Check sheet for the modelled part. Datum: model origin and axes. Units: mm. Face numbers are marked on the shaded views. A direction names the side the tool comes from. Give positions to 0.01 mm unless a question says otherwise; leave off trailing zeros. Order: outer loops, then holes, each group sorted by start corner. A loop starts at its lowest first (then second) coordinate and runs counter-clockwise, first axis right, second up.
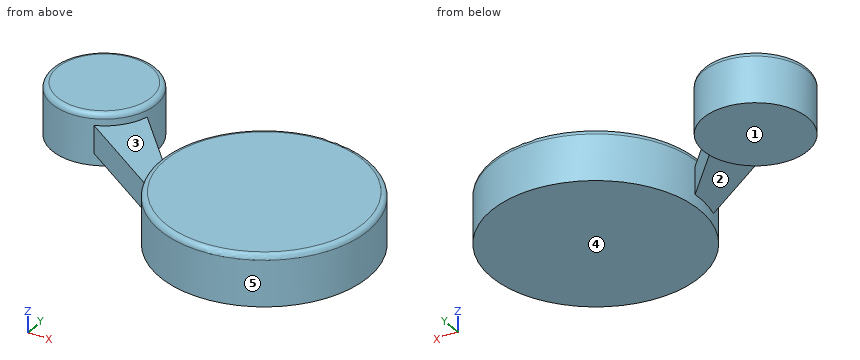
```python
from build123d import *

# Parameters (mm, degrees)
F0_R     = 101.6
F0_R_2   = 50.8
F1_DEPTH = 25
F2_R     = 5.08
F4_DEPTH = 13.5


with BuildPart() as f1:
    # F0 (on Top) → F1 (new body, symmetric)
    with BuildSketch(Plane.XY):
        with Locations((204.801934, 0)):
            Circle(F0_R)
        with Locations((0, 80.350283)):
            Circle(F0_R_2)
    extrude(amount=F1_DEPTH, both=True)

    # F2
    f2_edges = [f1.edges().sort_by_distance(p)[0] for p in [
        (-50.8, 80.350283, 25),
        (103.201934, 0, 25),
    ]]
    fillet(f2_edges, radius=F2_R)

    # F3 (on Top) → F4 (join, symmetric)
    with BuildSketch(Plane.XY):
        Polygon((10.487304, 110.720679), (17.449906, 34.354378), (178.083748, -74.550241), align=None)
    extrude(amount=F4_DEPTH, both=True)


solid = f1.part
```
(1) Cross-section at B-B on z = 6. Enter the section's corners in (x, y), then the cut area to 3 significant figures.
Response values:
outline: (19.06, 33.26) - (106.61, -26.09) arc R101.6 ccw (long way) to (103.51, 7.89) - (49.24, 67.88) arc R50.8 ccw (long way) to start
area: 43,600 mm2
(2) Cross-section at C-C on y = 0. Enter the section's corners in (x, z).
Response values:
outline: (68.12, -13.5) - (103.2, -13.5) - (103.2, -25) - (306.4, -25) - (306.4, 19.92) arc R5.08 ccw to (301.32, 25) - (108.28, 25) arc R5.08 ccw to (103.2, 19.92) - (103.2, 13.5) - (68.12, 13.5) - close
(3) Material ranges on L1, parallel to X at y = 89, z = -6; L2, parallel to Z at x = 77, y = -4; L3, parallel to X at y = 34.5, z = 11.5, recorded low to high.
Response values:
L1: x = -50.06 to 50.06, 155.8 to 253.81
L2: z = -13.5 to 13.5
L3: x = -21.87 to 79.44, 109.24 to 300.37
(4) Cross-section at D-D on z = -21. Enter the section's corners in (x, y).
Response values:
outline: circle Ø101.6 at (0, 80.35); circle Ø203.2 at (204.8, 0)
(5) Gauge pin test, flat ends, axial feed: pin 1 Ø3 at (y, z) = (76.5, 14.5) entering from +X; pin 2 Ø1 at (y, z) = (-5, -0.5) entering from -X; pin 3 Ø6 at (x, z) = (215, 5) entering from -Y. Record the tip position at first contact, or that the pin passes through.
Response values:
pin 1: stops at x = 273.34
pin 2: stops at x = 74.76
pin 3: stops at y = -101.34
(6) Cross-section at A-A on x = 0. Enter the section's corners in (y, z), then the cut area to 3 significant figures.
Response values:
outline: (29.55, -25) - (131.15, -25) - (131.15, 19.92) arc R5.08 ccw to (126.07, 25) - (34.63, 25) arc R5.08 ccw to (29.55, 19.92) - close
area: 5,070 mm2
(7) Release check for a two-part mould opening along X. For the marked faces 4 and 5 record: released by +X, released by -X, zero draft, split by the parting line, or undercut.
Response values:
face 4: zero draft
face 5: undercut
(8) Set-up check for the marked faces 1, 2 and 3: record each of +Z, -Z, +X, -X, +Y, -Y from which the full face is reachable in a straight line by a thin tool's end or side.
Response values:
face 1: -Z, +X, -X, +Y, -Y
face 2: -Z, -Y
face 3: +Z, -Y
